from build123d import *

# Parameters (mm, degrees)
SKETCH1_W = 12
SKETCH1_H = 53.690960396


with BuildPart() as part:
    # Sketch1 → Revolve1 (revolve)
    with BuildSketch(Plane(origin=(0, 0, 0), x_dir=(0, 0, -1), z_dir=(1, 0, 0)), mode=Mode.PRIVATE) as revolve1_sk:
        with BuildLine():
            Line((0, 8.5), (-24.7, 8.5))
            Line((-24.7, 8.5), (-24.7, 66))
            ThreePointArc((-24.7, 66), (-22.903230037, 76.118602871), (-17.732611951, 85))
            ThreePointArc((-17.732611951, 85), (-9.761601016, 91.587591953), (0, 95))
            Line((0, 95), (0, 8.5))
        make_face()
        with Locations((-9.145311229, 53.422633767)):
            Rectangle(SKETCH1_W, SKETCH1_H, mode=Mode.SUBTRACT)
    revolve(revolve1_sk.sketch.rotate(Axis((0, 0, 15.387931034), (0, 0, -1)), 90), axis=Axis((0, 0, 15.387931034), (0, 0, -1)))


solid = part.part
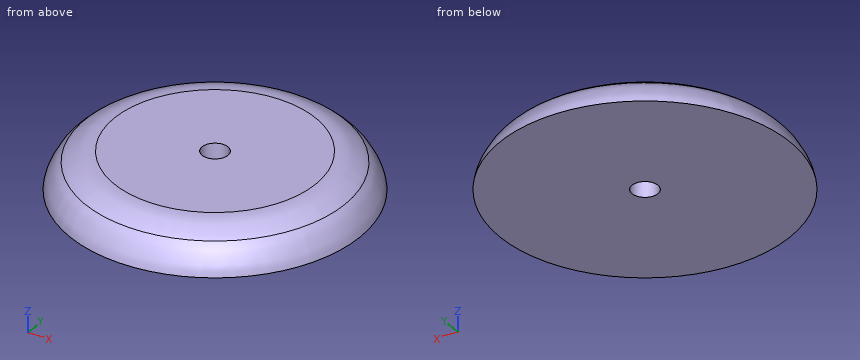
The listing builds one solid part. Answer for the finished solid, in the listing's coordinates (mm). Coordinates: 2 decimals unless noted, no trailing zeros. Write each loop counter-clockwise with the first axis right and the second up, starting at its lowest first coordinate (ties: lowest second). Pieces come first, ordered by that corner, then holes. Notation, with made-up numbers: (-5, 25) -> (-1, 25) arc R33 ccw to (-1, 61) -> close; hole circle Ø9 at (65.5, 27.5). An arc over 180 degrees is marked (long way). One line per question, with ' | ' between items.
1. Section C-C (z = 8.75) is taken. Determine the outline of the cut face in (x, y), and give its area (3 significant figures).
Verdict:
outline: circle Ø184.26 at (0, 0); circle Ø53.15 at (0, 0); hole circle Ø160.54 at (0, 0); hole circle Ø17 at (0, 0) | area: 8,420 mm^2
2. Section A-A (x = 0) is taken. Determine the outline of the cut face in (y, z), and give its area (3 significant figures).
Verdict:
outline: (-95, 0) -> (-8.5, 0) -> (-8.5, 24.7) -> (-66, 24.7) arc R29.39 ccw to (-85, 17.73) arc R29.33 ccw to start; (8.5, 0) -> (95, 0) arc R29.33 ccw to (85, 17.73) arc R29.39 ccw to (66, 24.7) -> (8.5, 24.7) -> close; hole (-80.27, 3.15) -> (-26.58, 3.15) -> (-26.58, 15.15) -> (-80.27, 15.15) -> close; hole (26.58, 3.15) -> (80.27, 3.15) -> (80.27, 15.15) -> (26.58, 15.15) -> close | area: 2,630 mm^2
3. Straight lines are drawn through the part: line 1 (Z direction, x = 12, y = -51); line 2 (X direction, y = -17, z = 8.5); line 3 (Y direction, x = 9.5, z = 3.5). For each, find the intervals that lie inside material, in ascending order.
Verdict:
line 1: z = 0 to 3.15, 15.15 to 24.7 | line 2: x = -90.68 to -78.45, -20.43 to 20.43, 78.45 to 90.68 | line 3: y = -93.74 to -79.7, -24.82 to 24.82, 79.7 to 93.74
4. Given pin 1 Ø4 at (x, z) = (60, 12.5) entering from +Y; pin 2 Ø1.5 at (x, z) = (76, 11.5) entering from -Y; pin 3 Ø1 at (x, z) = (26.5, 2.5) entering from -Y, each flat-ended and moving along its own axis, determine where each tip first touches the part or whether it passes through.
Verdict:
pin 1: stops at y = 69.36 | pin 2: stops at y = -50.62 | pin 3: stops at y = -90.89
